Can you work these out from the model? Positions are in its coordinate system, mm. A direction names the side the tool comes from. Coordinates: 2 decimals unless noted, no trailing zeros. Order: outer loops, then holes, each group sorted by start corner. A loop starts at its lowest first (then second) coordinate and runs counter-clockwise, first axis right, second up.
```python
from build123d import *

# Parameters (mm, degrees)
F0_W     = 2057.4
F0_H     = 990.6
F1_DEPTH = 939.8
F3_DEPTH = 876.3
F5_DEPTH = 127000
F7_DEPTH = 152.4


with BuildPart() as f1:
    # F0 (on Top) → F1 (new body)
    with BuildSketch(Plane.XY):
        Rectangle(F0_W, F0_H)
    extrude(amount=F1_DEPTH)

    # F2 (on Right) → F3 (cut, symmetric)
    with BuildSketch(Plane.YZ):
        Polygon((-495.3, 939.8), (-495.3, 533.4), (88.9, 533.4), (160.5592849599, 939.8), align=None)
    extrude(amount=F3_DEPTH, both=True, mode=Mode.SUBTRACT)

    # F4 (on Right) → F5 (cut, symmetric)
    with BuildSketch(Plane.YZ):
        Polygon((-495.3, 939.8), (-495.3, 609.6), (102.33611593, 609.6), (160.5592849599, 939.8), align=None)
    extrude(amount=F5_DEPTH, both=True, mode=Mode.SUBTRACT)

    # F6 (on face) → F7 (cut)
    with BuildSketch(Plane(origin=(0, 0, 0), x_dir=(1, 0, 0), z_dir=(0, 0, -1))):
        Polygon((977.9, 495.3), (-977.9, 495.3), (-977.9, 444.5), (-1028.7, 444.5), (-1028.7, -444.5), (-977.9, -444.5), (-977.9, -495.3), (977.9, -495.3), (977.9, -444.5), (1028.7, -444.5), (1028.7, 444.5), (977.9, 444.5), align=None)
    extrude(amount=-F7_DEPTH, mode=Mode.SUBTRACT)


solid = f1.part
```
1. Imagine slicing it at C-C on y = 326. Please give me the cut outline in (x, z).
Completed:
outline: (-1028.7, 152.4) - (1028.7, 152.4) - (1028.7, 939.8) - (-1028.7, 939.8) - close
2. Imagine slicing it at A-A on x = 57.5. Please give me the cut outline in (y, z), then the cut area to 3 significant figures.
Completed:
outline: (-495.3, 152.4) - (495.3, 152.4) - (495.3, 939.8) - (160.56, 939.8) - (88.9, 533.4) - (-495.3, 533.4) - close
area: 528,000 mm2
3. On a 3-axis mill with a long thin cutter (end or side, diameter ignored), from which of +Z, -Z, +X, -X, +Y, -Y can I reach the whole of each face in a straight line? I mean faces 4 (the flat face through (977.9, -470, 75)), 5 (the flat face through (12, -207, 533.4)), 6 (the flat face through (1004, -444.5, 75)), 7 (the flat face through (-1004, 470, 0)), 8 (the flat face through (954, -201, 609.6)). Say none if no direction works.
Completed:
face 4: -Z, +Y, -Y
face 5: +Z, -Y
face 6: -Z, +X, -X
face 7: -Z, +X, -X, +Y, -Y
face 8: +Z, +X, -X, -Y
4. Thinking about a two-plate mould opening in Y: for faces 1 (the flat face through (1003, 444.5, 75)), 2 (the flat face through (-1004, -470, 0)), 3 (the flat face through (-14, 495.3, 568)), which applies, pulls with the +Y half, pulls with the -Y half, needs draft (parallel to the pull), parting line crosses it, or undercut?
Completed:
face 1: undercut
face 2: needs draft
face 3: pulls with the +Y half
5. Please list where these lines run through material, in increasing order: probe 1 along Z at (x, y) = (-531.5, -74); probe 2 along Z at (x, y) = (-563.5, 267); probe 3 along Y at (x, z) = (-81.5, 772).
Completed:
probe 1: z = 152.4 to 533.4
probe 2: z = 152.4 to 939.8
probe 3: y = 130.97 to 495.3
6. Imagine slicing it at D-D on z = 768.5. Please give me the cut outline in (x, y), then the cut area to 3 significant figures.
Completed:
outline: (-1028.7, 130.35) - (1028.7, 130.35) - (1028.7, 495.3) - (-1028.7, 495.3) - close
area: 751,000 mm2
7. I'm going to push a flat-ended pin straight in: pin 1 (2 mm diameter, centred on x = -252, z = 539, fed in from -Y). Where does the tip first touch, or does it pass through?
Completed:
pin 1: stops at y = 89.71
8. Imagine slicing it at B-B on y = -2. Please give me the cut outline in (x, z), then the cut area to 3 significant figures.
Completed:
outline: (-1028.7, 152.4) - (1028.7, 152.4) - (1028.7, 609.6) - (876.3, 609.6) - (876.3, 533.4) - (-876.3, 533.4) - (-876.3, 609.6) - (-1028.7, 609.6) - close
area: 807,000 mm2
